Part model, mm, in its own coordinate system. Coordinates: 2 decimals unless noted, no trailing zeros. Loops run counter-clockwise (first coordinate to the right, second up) from the corner with the lowest first, then second, coordinate; pieces in that order, holes last. Notation, with made-up numbers: M 88,19 L 123,19 A22 cw 123,32 Z; hole C -17.5,79.5 d7. An arc over 180 degrees is marked long. Answer as a JSON object with one key per item and string values. Group by question number.
1. Mould opens along X. For faces 1 (the face through (-48.859, -38.797, 1.726)), 2 (the face through (47.24, 35.08, 1.73)), 3 (the face through (50, -1, 2)) say: released by +X, released by -X, zero draft, split by the parting line, or undercut.
2. Drill centre lines: L1, parallel to Y at x = -29, z = 1.7; L2, parallel to Y at x = -46.5, z = 2.1. Where is each one in solid material? Low to high.
3. Drop a flat-ended pin along its axis: pin 1 Ø1.9 at (x, y) = (-46.5, -36.5) entering from +Z. Give the stop position or say it passes through.
4. Saw through at B-B on x = 29. Write the cut outline in (y, z).
5. Saw through at A-A on y = -24.5. Write the cut outline in (x, z).
from build123d import *

# Parameters (mm, degrees)
SKETCH2_R           = 1.6
BOSS_EXTRUDE1_DEPTH = 3.5
SKETCH3_R           = 1.5
CUT_EXTRUDE1_DEPTH  = 8


with BuildPart() as part:
    # Sketch2 → Boss-Extrude1 (new body)
    with BuildSketch(Plane.XY):
        with BuildLine():
            Line((-46, -40), (46, -40))
            ThreePointArc((46, -40), (48.828427125, -38.828427125), (50, -36))
            Line((50, -36), (50, 36))
            ThreePointArc((50, 36), (48.828427125, 38.828427125), (46, 40))
            Line((46, 40), (-46, 40))
            ThreePointArc((-46, 40), (-48.828427125, 38.828427125), (-50, 36))
            Line((-50, 36), (-50, -36))
            ThreePointArc((-50, -36), (-48.828427125, -38.828427125), (-46, -40))
        make_face()
        with Locations((-46.5, 36.5)):
            Circle(SKETCH2_R, mode=Mode.SUBTRACT)
        with Locations((46.5, 36.5)):
            Circle(SKETCH2_R, mode=Mode.SUBTRACT)
        with Locations((-46.5, -36.5)):
            Circle(SKETCH2_R, mode=Mode.SUBTRACT)
        with Locations((46.5, -36.5)):
            Circle(SKETCH2_R, mode=Mode.SUBTRACT)
    extrude(amount=BOSS_EXTRUDE1_DEPTH)

    # Sketch3 → Cut-Extrude1 (cut)
    with BuildSketch(Plane.XY.offset(3.5)):
        with Locations((-29, 24.5)):
            Circle(SKETCH3_R)
        with Locations((-29, -24.5)):
            Circle(SKETCH3_R)
        with Locations((29, -24.5)):
            Circle(SKETCH3_R)
        with Locations((29, 24.5)):
            Circle(SKETCH3_R)
    extrude(amount=-CUT_EXTRUDE1_DEPTH, mode=Mode.SUBTRACT)


solid = part.part
Outcome:
{
 "1": {"face 1": "released by -X", "face 2": "undercut", "face 3": "released by +X"},
 "2": {"L1": "y = -40 to -26, -23 to 23, 26 to 40", "L2": "y = -39.97 to -38.1, -34.9 to 34.9, 38.1 to 39.97"},
 "3": {"pin 1": "passes through"},
 "4": {"outline": "M -40,0 L -26,0 L -26,3.5 L -40,3.5 Z; M -23,0 L 23,0 L 23,3.5 L -23,3.5 Z; M 26,0 L 40,0 L 40,3.5 L 26,3.5 Z"},
 "5": {"outline": "M -50,0 L -30.5,0 L -30.5,3.5 L -50,3.5 Z; M -27.5,0 L 27.5,0 L 27.5,3.5 L -27.5,3.5 Z; M 30.5,0 L 50,0 L 50,3.5 L 30.5,3.5 Z"}
}
